Input: part model. Units: mm. Frame: model coordinates. A direction names the side the tool comes from. Coordinates: 2 decimals unless noted, no trailing zeros. Write each loop counter-clockwise with the first axis right and the second up, starting at its lowest first coordinate (ties: lowest second). Pieces come first, ordered by that corner, then holes. Notation, with made-up numbers: (39, 63) - (73, 63) arc R24 cw to (73, 74) - close; hole circle Ø5 at (-28, 14). An arc over 180 degrees is marked (long way). Use CSV: the item, a comma, the result in double quotes.
```python
from build123d import *

# Parameters (mm, degrees)
SKETCH1_W               = 50
SKETCH1_H               = 34.11
BOSS_EXTRUDE1_DEPTH     = 20
SKETCH2_R               = 2
BOSS_EXTRUDE2_DEPTH     = 10
LPATTERN1_COUNT         = 3
LPATTERN1_PITCH         = 20
MIRROR1_COPY_1_SKETCH_R = 2
MIRROR1_COPY_1_DEPTH    = 10
MIRROR1_COPY_2_SKETCH_R = 2
MIRROR1_COPY_2_DEPTH    = 10
SKETCH3_R               = 8
SKETCH3_W               = 3
SKETCH3_H               = 30
CUT_EXTRUDE1_DEPTH      = 10


with BuildPart() as part:
    # Sketch1 → Boss-Extrude1 (new body)
    with BuildSketch(Plane(origin=(0, 0, 0), x_dir=(0, 0, -1), z_dir=(1, 0, 0))):
        with Locations((25, 17.055)):
            Rectangle(SKETCH1_W, SKETCH1_H)
    extrude(amount=BOSS_EXTRUDE1_DEPTH)

    # Sketch2 → Boss-Extrude2 (add)
    with BuildSketch(Plane.XY):
        with BuildLine():
            Line((20, 34.11), (23, 34.11))
            ThreePointArc((23, 34.11), (26, 37.11), (23, 40.11))
            Line((23, 40.11), (20, 40.11))
            Line((20, 40.11), (14, 34.11))
            Line((14, 34.11), (20, 34.11))
        make_face()
        with Locations((23, 37.11)):
            Circle(SKETCH2_R, mode=Mode.SUBTRACT)
    boss_extrude2 = extrude(amount=-BOSS_EXTRUDE2_DEPTH)

    # LPattern1: Boss-Extrude2 ×3
    with Locations(*[(0, 0, -i * LPATTERN1_PITCH) for i in range(1, LPATTERN1_COUNT)]):
        add(boss_extrude2)

    # Mirror1: Boss-Extrude2 across plane
    add(boss_extrude2.mirror(Plane.ZX.offset(17.055)))

    # Mirror1 copy 1 sketch → Mirror1 copy 1 (add)
    with BuildSketch(Plane(origin=(0, 34.11, -20), x_dir=(1, 0, 0), z_dir=(0, 0, 1))):
        with BuildLine():
            Line((20, -34.11), (23, -34.11))
            ThreePointArc((23, -34.11), (26, -37.11), (23, -40.11))
            Line((23, -40.11), (20, -40.11))
            Line((20, -40.11), (14, -34.11))
            Line((14, -34.11), (20, -34.11))
        make_face()
        with Locations((23, -37.11)):
            Circle(MIRROR1_COPY_1_SKETCH_R, mode=Mode.SUBTRACT)
    extrude(amount=-MIRROR1_COPY_1_DEPTH)

    # Mirror1 copy 2 sketch → Mirror1 copy 2 (add)
    with BuildSketch(Plane(origin=(0, 34.11, -40), x_dir=(1, 0, 0), z_dir=(0, 0, 1))):
        with BuildLine():
            Line((20, -34.11), (23, -34.11))
            ThreePointArc((23, -34.11), (26, -37.11), (23, -40.11))
            Line((23, -40.11), (20, -40.11))
            Line((20, -40.11), (14, -34.11))
            Line((14, -34.11), (20, -34.11))
        make_face()
        with Locations((23, -37.11)):
            Circle(MIRROR1_COPY_2_SKETCH_R, mode=Mode.SUBTRACT)
    extrude(amount=-MIRROR1_COPY_2_DEPTH)

    # Sketch3 → Cut-Extrude1 (cut)
    with BuildSketch(Plane.ZY):
        with Locations((-25, 17.055)):
            Circle(SKETCH3_R)
        with Locations((-39, 17.055)):
            Rectangle(SKETCH3_W, SKETCH3_H)
        with Locations((-11, 17.055)):
            Rectangle(SKETCH3_W, SKETCH3_H)
    extrude(amount=-CUT_EXTRUDE1_DEPTH, mode=Mode.SUBTRACT)


solid = part.part
```
(1) Reachability of faces 4 (the flat face through (8, 34.11, -25)), 5 (the flat face through (8, 0, -25)), 6 (the flat face through (20, -2, -30)), 7 (the flat face through (5, 32.055, -11)), 8 (the flat face through (20, 36, -30)) from +Z, -Z, +X, -X, +Y, -Y: full face, straight path, thin tool, end or side. Return the list, or none.
Check values:
face 4,"-X, +Y"
face 5,"-X, -Y"
face 6,"+X, -X, -Y"
face 7,"-X"
face 8,"+X, -X, +Y"
(2) Draft query along X for faces 1 (the flat face through (17.04, 37.15, -24.93)), 2 (the flat face through (5, 17, -12.5)), 3 (the cylindrical face through (21.4, -4.2, -44.9)). Return one class per face: pulls with the +X half, pulls with the -X half, needs draft (parallel to the pull), parting line crosses it, or undercut.
Check values:
face 1,"pulls with the -X half"
face 2,"needs draft"
face 3,"undercut"
(3) Cut plane D-D on y = 29.5. Return loops of the section in (x, z), and give its area (3 significant figures).
Check values:
outline,"(0, -50) - (20, -50) - (20, 0) - (0, 0) - (0, -9.5) - (10, -9.5) - (10, -12.5) - (0, -12.5) - (0, -37.5) - (10, -37.5) - (10, -40.5) - (0, -40.5) - close"
area,"940 mm^2"
(4) Cut plane C-C on x = 18.25. Return loops of the section in (y, z), and give its area (3 significant figures).
Check values:
outline,"(-4.25, -50) - (38.36, -50) - (38.36, -40) - (34.11, -40) - (34.11, -30) - (38.36, -30) - (38.36, -20) - (34.11, -20) - (34.11, -10) - (38.36, -10) - (38.36, 0) - (-4.25, 0) - (-4.25, -10) - (0, -10) - (0, -20) - (-4.25, -20) - (-4.25, -30) - (0, -30) - (0, -40) - (-4.25, -40) - close"
area,"1,960 mm^2"
(5) Ray query, probe 1 along Z at (x, y) = (7.75, 32); probe 2 along Z at (x, y) = (18, 34.5); probe 3 along Y at (x, z) = (23, -45). Return the intervals inside material, ascending. Write a range as from..to.
Check values:
probe 1,"-50..-40.5, -37.5..-12.5, -9.5..0"
probe 2,"-50..-40, -30..-20, -10..0"
probe 3,"-6..-5, -1..0, 34.11..35.11, 39.11..40.11"
(6) Cut plane A-A on y = 37.11. Return loops of the section in (x, z).
Check values:
outline,"(17, -50) - (21, -50) - (21, -40) - (17, -40) - close; (17, -30) - (21, -30) - (21, -20) - (17, -20) - close; (17, -10) - (21, -10) - (21, 0) - (17, 0) - close; (25, -50) - (26, -50) - (26, -40) - (25, -40) - close; (25, -30) - (26, -30) - (26, -20) - (25, -20) - close; (25, -10) - (26, -10) - (26, 0) - (25, 0) - close"
(7) Cut plane B-B on z = -25. Return loops of the section in (x, y) (3 decimals).
Check values:
outline,"(0, 0) - (14, 0) - (20, -6) - (23, -6) arc R3 ccw to (23, 0) - (20, 0) - (20, 34.11) - (23, 34.11) arc R3 ccw to (23, 40.11) - (20, 40.11) - (14, 34.11) - (0, 34.11) - (0, 25.055) - (10, 25.055) - (10, 9.055) - (0, 9.055) - close; hole circle Ø4 at (23, -3); hole circle Ø4 at (23, 37.11)"
(8) Pin query (flat end, axial travel): pin 1 Ø1 at (y, z) = (9.5, -17.5) entering from +X; pin 2 Ø0.9 at (y, z) = (20.5, -11.5) entering from -X; pin 3 Ø6 at (x, z) = (5.5, -19.5) entering from +Y. Return the tip coordinate at first contact, or that it passes through.
Check values:
pin 1,"x = 20"
pin 2,"x = 10"
pin 3,"y = 34.11"
